```python
from build123d import *

# Parameters (mm, degrees)
BROCA_DE_ROSQUEAR_PARA_TARRAXA_DE_M41_D     = 3.3
BROCA_DE_ROSQUEAR_PARA_TARRAXA_DE_M41_DEPTH = 6.008579979
BROCA_DE_ROSQUEAR_PARA_TARRAXA_DE_M41_TIP   = 0.991420021


with BuildPart() as part:
    # Esboço1 → Revolução1 (revolve)
    with BuildSketch(Plane.XY, mode=Mode.PRIVATE) as revolu_o1_sk:
        Polygon((-2, 0), (-3.5, 0), (-3, -0.5), (-3, -0.75), (-4.25, -0.75), (-4.25, -1.95), (-2.95, -1.95), (-2.95, -7.25), (-2.45, -7.75), (0, -7.75), (0, -2), (-1.133974596, -2), (-2, -1.5), align=None)
    revolve(revolu_o1_sk.sketch.rotate(Axis((0, -2, 0), (0, -1, 0)), 270), axis=Axis((0, -2, 0), (0, -1, 0)))

    # Broca de rosquear para tarraxa de M41
    with Locations(Plane(origin=(0, 0, 0), x_dir=(1, 0, 0), z_dir=(0, 1, 0))):
        with Locations((0, 0)):
            Hole(BROCA_DE_ROSQUEAR_PARA_TARRAXA_DE_M41_D / 2, depth=BROCA_DE_ROSQUEAR_PARA_TARRAXA_DE_M41_DEPTH)
            with Locations((0, 0, -(BROCA_DE_ROSQUEAR_PARA_TARRAXA_DE_M41_DEPTH + BROCA_DE_ROSQUEAR_PARA_TARRAXA_DE_M41_TIP / 2))):  # 118° drill point
                Cone(0, BROCA_DE_ROSQUEAR_PARA_TARRAXA_DE_M41_D / 2, BROCA_DE_ROSQUEAR_PARA_TARRAXA_DE_M41_TIP, mode=Mode.SUBTRACT)


solid = part.part
```
Here's how the part is built. I have some questions about the finished solid (model axes, mm). A direction names the side the tool comes from. Round coordinates to 2 decimals unless told otherwise and drop trailing zeros. Loops run counter-clockwise (first coordinate to the right, second up) from the corner with the lowest first, then second, coordinate; pieces in that order, holes last.
1. If I drill on probe 1 along X at (y, z) = (-0.6, 0); probe 2 along X at (y, z) = (-5, -1); probe 3 along Y at (x, z) = (4, 1.25), over which ranges is the centre line in solid material (lowest first)?
Answers:
probe 1: x = -3 to -2, 2 to 3
probe 2: x = -2.78 to -1.31, 1.31 to 2.78
probe 3: y = -1.95 to -0.75
2. Suppose I cut it at A-A, the plane y = -5.5. Please give me the cut outline in (x, z), and give its area (3 significant figures).
Answers:
outline: circle Ø5.9 at (0, 0); hole circle Ø3.3 at (0, 0)
area: 18.8 mm2
3. For faces 5 (the face through (1.216, -3.885, -1.115)), 6 (the face through (-3, -0.75, -1)), 7 (the face through (0, -7.75, 0)), which set-ups out of +Z, -Z, +X, -X, +Y, -Y let a thin tool reach every point of the face, with its end or its side?
Answers:
face 5: +Y
face 6: none
face 7: +Z, -Z, +X, -X, -Y
4. Thinking about a two-plate mould opening in Z: for faces 1 (the face through (2, -1, 0)), 2 (the face through (1, -1.95, -3)), 3 (the face through (2.88, -4.64, -0.64)), 4 (the face through (0, -7, 0)), which applies, released by +Z, released by -Z, zero draft, split by the parting line, or undercut?
Answers:
face 1: undercut
face 2: zero draft
face 3: split by the parting line
face 4: undercut
5. Will these pins go through, and if not, where does the flat tip stop? pin 1 (3 mm diameter, centred on x = 0, z = 0, fed in from +Y); pin 2 (1 mm diameter, centred on y = -7, z = 1, fed in from -X); pin 3 (2 mm diameter, centred on y = -6, z = 2, fed in from -X).
Answers:
pin 1: stops at y = -6.1
pin 2: stops at x = -2.91
pin 3: stops at x = -2.78
